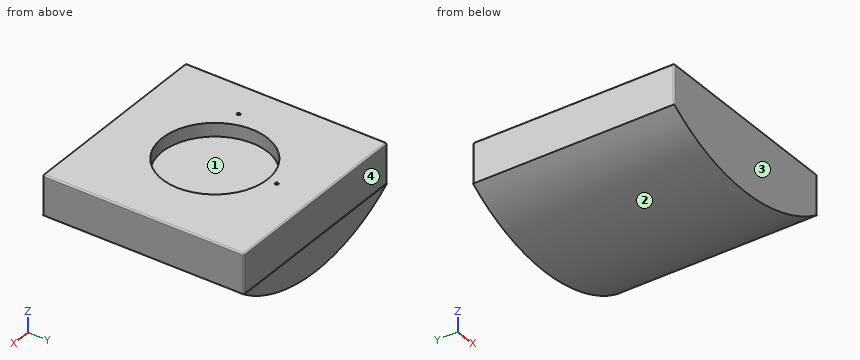
from build123d import *

# Parameters (mm, degrees)
SKETCH1_W                       = 150
SKETCH1_H                       = 150
BOSS_EXTRUDE1_DEPTH             = 30
FILLET1_R                       = 1
SKETCH2_R                       = 39.25
CUT_EXTRUDE4_DEPTH              = 10
TAP_DRILL_FOR_M6X1_0_TAP1_D     = 5
TAP_DRILL_FOR_M6X1_0_TAP1_DEPTH = 12
TAP_DRILL_FOR_M6X1_0_TAP1_TIP   = 1.502151548
BOSS_EXTRUDE2_DEPTH             = 150
TAP_DRILL_FOR_M3X0_5_TAP3_D     = 2.5
TAP_DRILL_FOR_M3X0_5_TAP3_DEPTH = 10
TAP_DRILL_FOR_M3X0_5_TAP3_TIP   = 0.751075774


with BuildPart() as part:
    # Sketch1 → Boss-Extrude1 (new body)
    with BuildSketch(Plane.XY):
        Rectangle(SKETCH1_W, SKETCH1_H)
    extrude(amount=-BOSS_EXTRUDE1_DEPTH)

    # Fillet1
    fillet1_edges = [part.edges().sort_by_distance(p)[0] for p in [
        (0, 75, -30),
        (-75, 0, 0),
        (0, 75, 0),
        (75, 0, 0),
        (0, -75, 0),
        (-75, -75, -15),
        (-75, 75, -15),
        (75, 75, -15),
        (75, -75, -15),
        (75, 0, -30),
    ]]
    fillet(fillet1_edges, radius=FILLET1_R)

    # Sketch2 → Cut-Extrude4 (cut)
    with BuildSketch(Plane.XY):
        Circle(SKETCH2_R)
    extrude(amount=-CUT_EXTRUDE4_DEPTH, mode=Mode.SUBTRACT)

    # Tap Drill for M6x1.0 Tap1
    with Locations(Plane(origin=(0, 0, -30), x_dir=(-1, 0, 0), z_dir=(0, 0, -1))):
        with Locations((-61.528492196, 5.588819372), (-61.436853723, -13.886414682), (66.990456482, 6.193550496), (67.082094955, -13.281683558)):
            Hole(TAP_DRILL_FOR_M6X1_0_TAP1_D / 2, depth=TAP_DRILL_FOR_M6X1_0_TAP1_DEPTH)
            with Locations((0, 0, -(TAP_DRILL_FOR_M6X1_0_TAP1_DEPTH + TAP_DRILL_FOR_M6X1_0_TAP1_TIP / 2))):  # 118° drill point
                Cone(0, TAP_DRILL_FOR_M6X1_0_TAP1_D / 2, TAP_DRILL_FOR_M6X1_0_TAP1_TIP, mode=Mode.SUBTRACT)

    # Sketch11 → Boss-Extrude2 (add)
    with BuildSketch(Plane.XZ.offset(75)):
        with BuildLine():
            Line((-75, -30), (74.707106781, -29.707106781))
            ThreePointArc((74.707106781, -29.707106781), (-0.100328988, -53.42574699), (-75, -30))
        make_face()
    extrude(amount=-BOSS_EXTRUDE2_DEPTH)

    # Tap Drill for M3x0.5 Tap3
    with Locations(Plane.XY):
        with Locations((0.496213053, 46.5), (-48.237547134, -16.547252974)):
            Hole(TAP_DRILL_FOR_M3X0_5_TAP3_D / 2, depth=TAP_DRILL_FOR_M3X0_5_TAP3_DEPTH)
            with Locations((0, 0, -(TAP_DRILL_FOR_M3X0_5_TAP3_DEPTH + TAP_DRILL_FOR_M3X0_5_TAP3_TIP / 2))):  # 118° drill point
                Cone(0, TAP_DRILL_FOR_M3X0_5_TAP3_D / 2, TAP_DRILL_FOR_M3X0_5_TAP3_TIP, mode=Mode.SUBTRACT)


solid = part.part
Geometry: final body of the model. Coordinates: model frame, mm. Face numbers are marked on the shaded views. Round coordinates to 2 decimals unless told otherwise and drop trailing zeros. Loops run counter-clockwise (first coordinate to the right, second up) from the corner with the lowest first, then second, coordinate; pieces in that order, holes last. Notation, with made-up numbers: M 57,66.25 L 95,66.25 A24 ccw 95,77.25 Z; hole C 81.25,82 d7. An arc over 180 degrees is marked long. Put each result on its own line as item: value. Start each with the question number.
(1) Section query D-D (x = -10.5). Return loops of the section in (y, z), then the cut area to 3 significant figures.
(2) Section query C-C (y = 0). Return loops of the section in (x, z).
(3) Material intervals for line 1 along X through (y, z) = (6, -24); line 2 along X through (y, z) = (46, -3); line 3 along Y through (x, z) = (10, -8.5), sorted ascending. Write a range as [from, to].
(4) Draft query along Y for the marked faces 1, 2, 3 and 4. Return one class per face: +Y half, -Y half, draft (parallel to the pull), parting line (faces both ways), or undercut.
(5) Section query B-B (x = 35). Return loops of the section in (y, z), then the cut area to 3 significant figures.
(6) Section query A-A (y = -50). Return loops of the section in (x, z), then the cut area to 3 significant figures.
(7) Contact query for flat-ended pins moving along their axis: pin 1 Ø1 at (y, z) = (0.5, -35.5) entering from -X; pin 2 Ø2 at (x, y) = (0.5, 46.5) entering from +Z; pin 3 Ø4 at (x, y) = (-66.99, 6.19) entering from -Z. Output: stop coordinate, or through.
Findings below:
1. outline: M -75,-53.03 L 75,-53.03 L 75,-29.87 L 74.49,-29.87 A1 ccw 75,-29 L 75,-1 A1 ccw 74,0 L 37.82,0 L 37.82,-10 L -37.82,-10 L -37.82,0 L -74,0 A1 ccw -75,-1 Z
1. area: 7,200 mm2
2. outline: M -75,-30 A130.64 ccw 74.42,-29.91 A1 ccw 75,-29 L 75,-1 A1 ccw 74,0 L 39.25,0 L 39.25,-10 L -39.25,-10 L -39.25,0 L -74,0 A1 ccw -75,-1 Z
3. line 1: x = [-75, -69.48], [-64.5, 59.06], [63.99, 75]
3. line 2: x = [-75, -0.65], [1.64, 75]
3. line 3: y = [-75, -37.95], [37.95, 75]
4. face 1: undercut
4. face 2: draft
4. face 3: -Y half
4. face 4: +Y half
5. outline: M -75,-48.55 L 75,-48.55 L 75,-29.78 L 74.62,-29.78 A1 ccw 75,-29 L 75,-1 A1 ccw 74,0 L 17.76,0 L 17.76,-10 L -17.76,-10 L -17.76,0 L -74,0 A1 ccw -75,-1 Z
5. area: 6,930 mm2
6. outline: M -75,-30 A130.64 ccw 74.42,-29.91 A1 ccw 75,-29 L 75,-1 A1 ccw 74,0 L -74,0 A1 ccw -75,-1 Z
6. area: 6,880 mm2
7. pin 1: stops at x = -67.25
7. pin 2: stops at z = -10.15
7. pin 3: stops at z = -36.32
